Autodesk Inventor part; units mm, degrees
ref_plane "YZ Plane" through (0, 0, 0) normal (1, 0, 0) x (0, 1, 0)
ref_plane "XZ Plane" through (0, 0, 0) normal (0, 1, 0) x (-1, 0, 0)
ref_plane "XY Plane" through (0, 0, 0) normal (0, 0, 1) x (1, 0, 0)
sketch "Sketch1" plane through (0, 0, 0) normal (0, 0, 1) x (1, 0, 0)
  arc A0 (32.6355, 29.9298) -> (29.3759, 33.1607) centre (29.5384, 30.0649) ccw
  arc A1 (27.8274, -32.2191) -> (30.1546, -26.93) centre (30.0194, -30.0271) ccw
  arc A2 (32.4933, 26.671) -> (34.0351, 30.2371) centre (29.5384, 30.0649) ccw
  arc A3 (26.8375, -33.2091) -> (34.5127, -29.7804) centre (30.0194, -30.0271) ccw
  line L0 (-29.9673, 30.0452) -> (-33.1472, 26.8653)
  line L1 (-29.9673, 30.0452) -> (-25.4702, 30.0452) construction
  line L2 (-29.9673, 30.0452) -> (-21.8579, 30.471)
  line L3 (30.0194, -30.0271) -> (30.3698, -21.9984)
  line L4 (30.0194, -30.0271) -> (26.8375, -33.2091)
  circle A4 centre (0, 0) radius 37.5
  arc A5 (34.5127, -29.7804) -> (34.0351, 30.2371) centre (-61.1139, -0.5306) ccw
  arc A6 (29.3158, 34.5594) -> (-29.9754, 34.5423) centre (-0.3022, -60.9538) ccw
  line L5 (18.5473, 32.5922) -> (29.3759, 33.1607)
  line L6 (32.1704, 19.2696) -> (32.6355, 29.9298)
  arc A7 (29.3158, 34.5594) -> (26.1185, 32.9896) centre (29.5384, 30.0649) ccw
  arc A8 (34.0351, 30.2371) -> (29.3158, 34.5594) centre (29.5384, 30.0649) ccw
  arc A9 (-29.9754, 34.5423) -> (-33.1472, 26.8653) centre (-29.9673, 30.0452) ccw
  arc A10 (-26.8454, 30.2091) -> (-32.1778, 27.8347) centre (-29.9673, 30.0452) ccw
  dimension "d0" = 6.2
  dimension "d1" = 6.2
  dimension "d6" = 9
  dimension "d7" = 9
  dimension "d8" = 135
  dimension "d9" = 75
  dimension "d11" = 100
  dimension "d12" = 100
extrude "Extrusion1" add sketch "Sketch1" along normal blind 75 contours A0 L5 A7 A8 A2 L6 | A2 A5 A3 L4 A1 L3 A4 L6 | L5 A4 L2 A10 L0 A9 A6 A7
properties part number "Cage60mm-2sides-InnerD75mm-L75mm"
Geometry: final body of the model. Coordinates: model frame, mm. A direction names the side the tool comes from. Coordinates: 2 decimals unless noted, no trailing zeros. Loops run counter-clockwise (first coordinate to the right, second up) from the corner with the lowest first, then second, coordinate; pieces in that order, holes last. Notation, with made-up numbers: (39, -37.5) -> (53, -37.5) arc R26 cw to (53, 0.5) -> close; hole circle Ø5 at (-10.75, -31.75). An arc over 180 degrees is marked (long way). Use a Markdown table: item, result. Add a question column.
(1) Line query: line 1 along X through (y, z) = (29, 41.5); line 2 along Y through (x, z) = (-30.5, 15); line 3 along X through (y, z) = (31.5, 71). Output: solid intervals per line, ascending.
(2) Access query for faces 4 (the cylindrical face through (31.695, 32.292, 36.975)), 5 (the flat face through (-24.39, 30.34, 36.98)), 6 (the flat face through (30.26, -24.5, 36.98)). Directions: +Z, -Z, +X, -X, +Y, -Y. A direction counts if a zero-diameter tool reaches every point of the face in a straight line with its end or side. Return the directions, or none.
(3) Pin query (flat end, axial travel): pin 1 Ø3 at (y, z) = (10.5, 40) entering from -X; pin 2 Ø3 at (x, z) = (-1, 14) entering from -Y; pin 3 Ø5 at (x, z) = (3.5, 27) entering from -Y; pin 4 Ø3.5 at (x, y) = (30.02, -30.03) entering from -Z. Return the tip coordinate at first contact, or that it passes through.
(4) Section query B-B, the plane x = 2. Return loops of the section in (y, z).
(5) Mould query, pull axis X, two halves, no side actions, for faces 1 (the cylindrical face through (37.476, -1.329, 36.975)), 2 (the flat face through (23.886, 32.872, 36.975)), 3 (the flat face through (16, 35, 75)). Classes: pulls with the +X half, pulls with the -X half, needs draft (parallel to the pull), parting line crosses it, or undercut.
(6) Section query A-A, the plane z = 20. Return loops of the section in (x, y), plus the area to 3 significant figures.
(7) Section query C-C, the plane y = 8. Return loops of the section in (x, z), plus the area to 3 significant figures.
Answer:
| question | item | result |
|---|---|---|
| 1 | line 1 | x = -34.34 to -32.91, 32.59 to 34.43 |
| 1 | line 2 | y = 33.13 to 34.51 |
| 1 | line 3 | x = -34.22 to -32.73, -27.2 to -20.35, 32.29 to 33.8 |
| 2 | face 4 | +Z, -Z |
| 2 | face 5 | +Z, -Z, -Y |
| 2 | face 6 | +Z, -Z, -X |
| 3 | pin 1 | stops at x = 35.53 |
| 3 | pin 2 | stops at y = 37.42 |
| 3 | pin 3 | stops at y = 37.02 |
| 3 | pin 4 | passes through |
| 4 | outline | (37.45, 0) -> (39.02, 0) -> (39.02, 75) -> (37.45, 75) -> close |
| 5 | face 1 | pulls with the -X half |
| 5 | face 2 | undercut |
| 5 | face 3 | needs draft |
| 6 | outline | (-33.15, 26.87) -> (-32.18, 27.83) arc R3.13 cw (long way) to (-26.85, 30.21) -> (-21.86, 30.47) arc R37.5 cw to (18.55, 32.59) -> (29.38, 33.16) arc R3.1 cw to (32.64, 29.93) -> (32.17, 19.27) arc R37.5 cw to (30.37, -22) -> (30.15, -26.93) arc R3.1 cw (long way) to (27.83, -32.22) -> (26.84, -33.21) arc R4.5 ccw to (34.51, -29.78) arc R100 ccw to (34.04, 30.24) arc R4.5 ccw to (29.32, 34.56) arc R100 ccw to (-29.98, 34.54) arc R4.5 ccw to start |
| 6 | area | 398 mm^2 |
| 7 | outline | (36.64, 0) -> (38.52, 0) -> (38.52, 75) -> (36.64, 75) -> close |
| 7 | area | 141 mm^2 |
